Can you work these out from the drawing? Everything is in mm from the part's minimum corner. Round coordinates to 2 decimals unless told otherwise and drop trailing zeros. Write each loop counter-clockwise with the first axis right and the second up, starting at its lowest first coordinate (ties: lowest second). Pieces come first, ordered by that corner, then holes. Notation, with made-up numbers: (48.5, 53) - (71.5, 53) arc R24 cw to (71.5, 71) - close; hole circle Ø4 at (68.5, 34.5). An arc over 180 degrees is marked (long way). One line per item, written item: value. Start each with the question number.
(1) I want a section at A-A on x = 2.6. List the corners of the cut face in (y, z) for me.
(2) If I drill on L1, parallel to Z at x = 2.25, y = 0.2; L2, parallel to Z at x = 2.75, y = 0.7; L3, parallel to X at y = 0.55, z = 5.25, over which ranges is the centre line in solid material (lowest first)? Write a range as from..to.
(3) Thinking about a two-plate mould opening in Z: for the marked faces 1, 2 and 3, which applies, +Z half, -Z half, draft (parallel to the pull), parting line (faces both ways), or undercut?
(4) I want a section at C-C on x = 1.5. List the corners of the cut face in (y, z) for me (1 decimal).
(5) I want a section at B-B on y = 0.4. List the corners of the cut face in (x, z) for me (1 decimal).
(6) I want a section at D-D on z = 1.5. List the corners of the cut face in (x, y) for me.
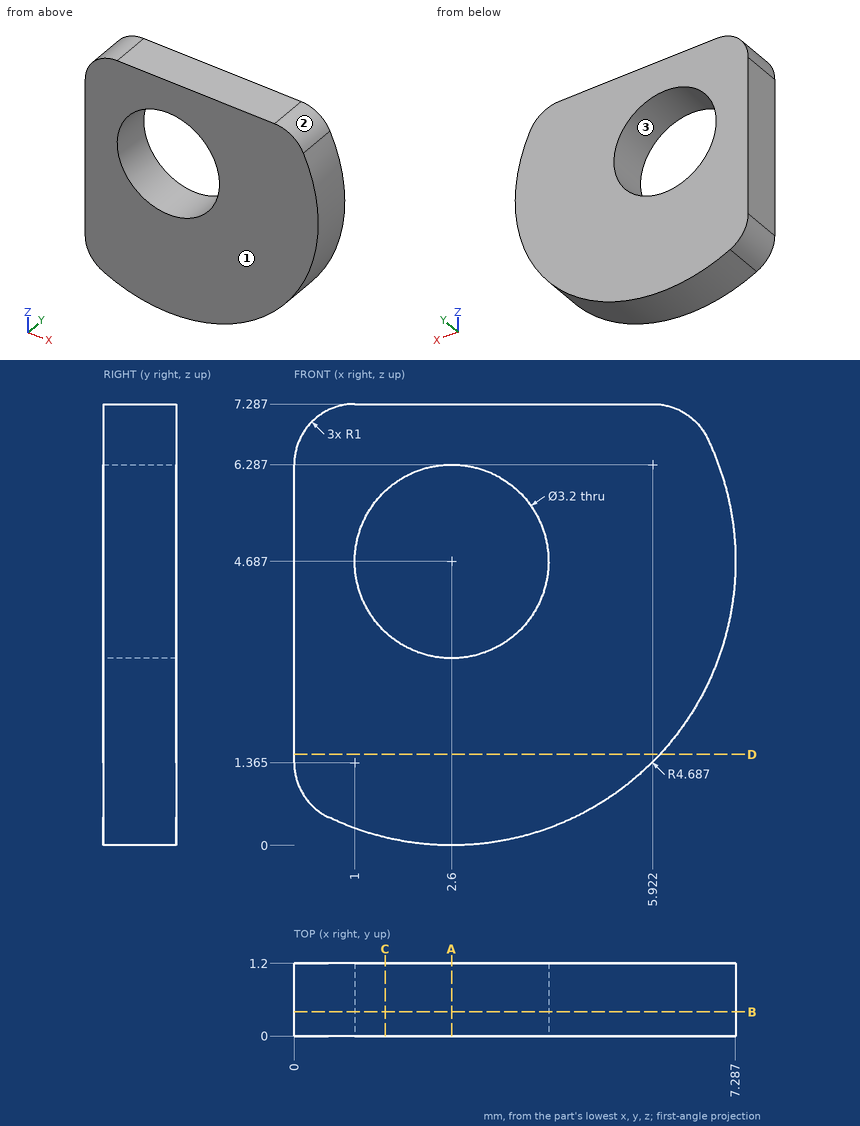
Established:
1. outline: (0, 0) - (1.2, 0) - (1.2, 3.09) - (0, 3.09) - close; (0, 6.29) - (1.2, 6.29) - (1.2, 7.29) - (0, 7.29) - close
2. L1: 0.01..3.13, 6.25..7.29
2. L2: 0..3.09, 6.28..7.29
2. L3: 0..1.1, 4.1..7.25
3. face 1: draft
3. face 2: +Z half
3. face 3: undercut
4. outline: (0, 0.1) - (1.2, 0.1) - (1.2, 3.5) - (0, 3.5) - close; (0, 5.8) - (1.2, 5.8) - (1.2, 7.3) - (0, 7.3) - close
5. outline: (0, 1.4) arc R1 ccw to (0.6, 0.5) arc R4.7 ccw to (6.8, 6.7) arc R1 ccw to (5.9, 7.3) - (1, 7.3) arc R1 ccw to (0, 6.3) - close; hole circle Ø3.2 at (2.6, 4.7)
6. outline: (0, 0) - (6.04, 0) - (6.04, 1.2) - (0, 1.2) - close
